from build123d import *

# Parameters (mm, degrees)
IZIM1_R                     = 10
IZIM1_R_2                   = 1.5
IZIM1_R_3                   = 4
Y_KSEKLIK_EKSTR_ZYON1_DEPTH = 5
IZIM2_R                     = 1.2
KES_EKSTR_ZYON1_DEPTH       = 10


with BuildPart() as part:
    # Çizim1 → Yükseklik-Ekstrüzyon1 (new body)
    # profile 1 of 3: a face of its own
    with BuildSketch(Plane.XY):
        Circle(IZIM1_R)
        Circle(IZIM1_R_2, mode=Mode.SUBTRACT)
    # profile 2 of 3: a face of its own
    with BuildSketch(Plane.XY):
        with BuildLine():
            Line((-3.899984172, 27.888888889), (-9.74996043, 2.222222222))
            ThreePointArc((-9.74996043, 2.222222222), (0, 10), (9.74996043, 2.222222222))
            Line((9.74996043, 2.222222222), (3.899984172, 27.888888889))
            ThreePointArc((3.899984172, 27.888888889), (3.974917401, 27.447248986), (4, 27))
            ThreePointArc((4, 27), (-0.447248986, 23.025082599), (-3.899984172, 27.888888889))
        make_face()
    # profile 3 of 3: a face of its own
    with BuildSketch(Plane.XY):
        with Locations((0, 27)):
            Circle(IZIM1_R_3)
        with Locations((0, 27)):
            Circle(IZIM1_R_2, mode=Mode.SUBTRACT)
    extrude(amount=Y_KSEKLIK_EKSTR_ZYON1_DEPTH)

    # Çizim2 → Kes-Ekstrüzyon1 (cut)
    with BuildSketch(Plane.XY.offset(5)):
        with Locations((0, 7)):
            Circle(IZIM2_R)
        with Locations((-7, 0)):
            Circle(IZIM2_R)
        with Locations((0, -7)):
            Circle(IZIM2_R)
        with Locations((7, 0)):
            Circle(IZIM2_R)
    extrude(amount=-KES_EKSTR_ZYON1_DEPTH, mode=Mode.SUBTRACT)


solid = part.part
Design review of the part built by this model. Coordinates are the model's own, in mm. Round coordinates to 2 decimals unless told otherwise and drop trailing zeros. Loops run counter-clockwise (first coordinate to the right, second up) from the corner with the lowest first, then second, coordinate; pieces in that order, holes last. Notation, with made-up numbers: (-37, 63.5) - (5, 63.5) arc R23 cw to (5, 95.5) - close; hole circle Ø2 at (34, -8). An arc over 180 degrees is marked (long way). One line per item, written item: value. Start each with the question number.
1) Consider section D-D on x = 0. Give the boundary of the cut face in (y, z), then the cut area to 3 significant figures.
2) Consider section B-B on x = -7.5. Give the boundary of the cut face in (y, z), then the cut area to 3 significant figures.
3) To check wall thickness, follow L1, parallel to Y at x = 0, z = 2.7; L2, parallel to Y at x = -1, z = 4.05; L3, parallel to X at y = 2, z = 2. State the ranges of each line that lie inside material, in increasing order. Write a range as from..to.
4) Insertion check: pin 1 Ø3 at (y, z) = (4.5, 1) entering from +X; pin 2 Ø1.5 at (x, z) = (3, 3.5) entering from -Y. Each pin has a flat end and moves straight along its axis. Give the tip position at first contact, or say it passes through.
5) Consider section A-A on z = 0.9. Give the boundary of the cut face in (x, y), then the cut area to 3 significant figures.
6) Consider section C-C on y = 7. Give the boundary of the cut face in (x, z).
Reported:
1. outline: (-10, 0) - (-8.2, 0) - (-8.2, 5) - (-10, 5) - close; (-5.8, 0) - (-1.5, 0) - (-1.5, 5) - (-5.8, 5) - close; (1.5, 0) - (5.8, 0) - (5.8, 5) - (1.5, 5) - close; (8.2, 0) - (25.5, 0) - (25.5, 5) - (8.2, 5) - close; (28.5, 0) - (31, 0) - (31, 5) - (28.5, 5) - close
1. area: 151 mm^2
2. outline: (-6.61, 0) - (-1.09, 0) - (-1.09, 5) - (-6.61, 5) - close; (1.09, 0) - (12.09, 0) - (12.09, 5) - (1.09, 5) - close
2. area: 82.6 mm^2
3. L1: y = -10..-8.2, -5.8..-1.5, 1.5..5.8, 8.2..25.5, 28.5..31
3. L2: y = -9.95..-7.66, -6.34..-1.12, 1.12..6.34, 7.66..25.88, 28.12..30.87
3. L3: x = -9.8..9.8
4. pin 1: stops at x = 9.57
4. pin 2: stops at y = -9.74
5. outline: (-9.75, 2.22) arc R10 ccw (long way) to (9.75, 2.22) - (3.9, 27.89) arc R4 ccw to (-3.9, 27.89) - close; hole circle Ø2.4 at (-7, 0); hole circle Ø3 at (0, 0); hole circle Ø3 at (0, 27); hole circle Ø2.4 at (0, -7); hole circle Ø2.4 at (0, 7); hole circle Ø2.4 at (7, 0)
5. area: 537 mm^2
6. outline: (-8.66, 0) - (-1.2, 0) - (-1.2, 5) - (-8.66, 5) - close; (1.2, 0) - (8.66, 0) - (8.66, 5) - (1.2, 5) - close
